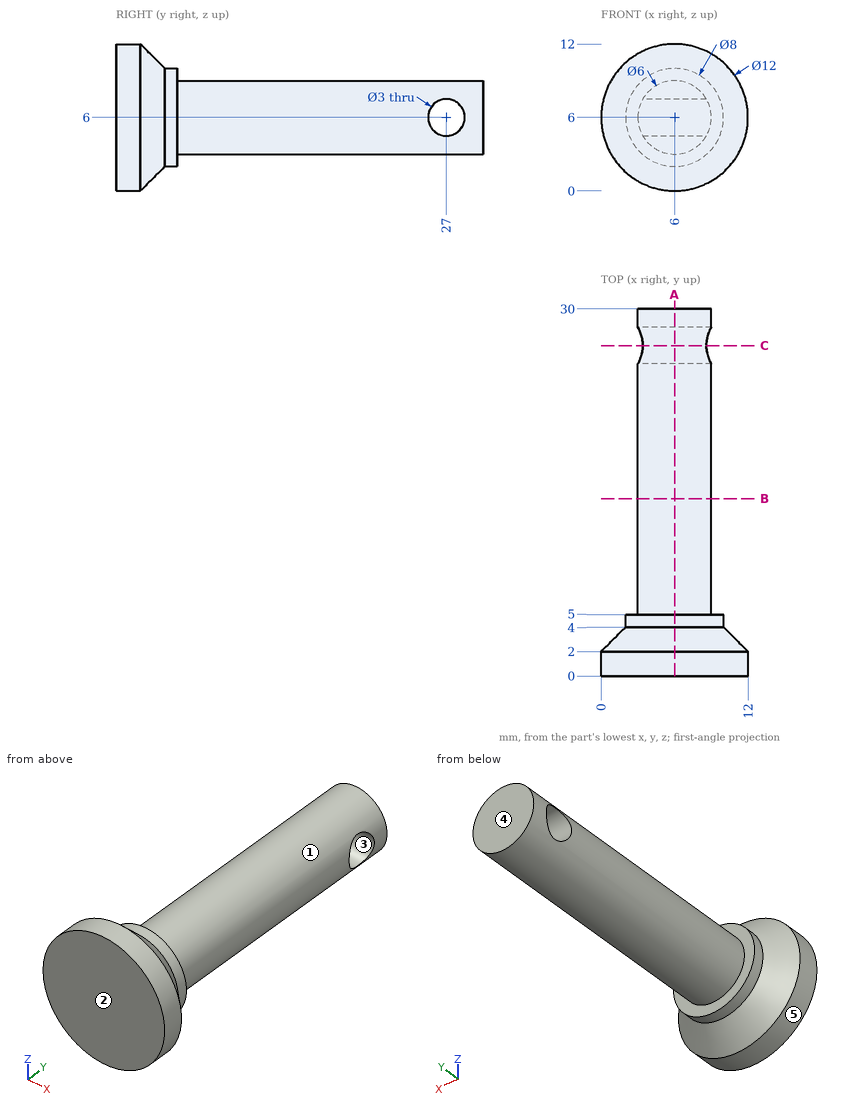
Here's the drawing with two shaded views (mm, measured from the low corner). I have some questions. A direction names the side the tool comes from. Coordinates: 2 decimals unless noted, no trailing zeros. Loops run counter-clockwise (first coordinate to the right, second up) from the corner with the lowest first, then second, coordinate; pieces in that order, holes last. Notation, with made-up numbers: (27, -27.5) - (42, -27.5) arc R22 cw to (42, -13.5) - close; hole circle Ø5 at (5, -31). An arc over 180 degrees is marked (long way). Answer as CSV lines item,"result". Start each with the question number.
1) Suppose I cut it at A-A (x = 6). Please give me the cut outline in (y, z).
2) Which directions (+Z, -Z, +X, -X, +Y, -Y) give clear straight access to the entire face, cutting with the end or side of a thin tool? Please do the marked faces 1 and 2.
3) Suppose I cut it at B-B (y = 14.5). Please give me the cut outline in (x, z).
4) Thinking about a two-plate mould opening in Z: for the marked faces 3, 4 and 5, which applies, pulls with the +Z half, pulls with the -Z half, needs draft (parallel to the pull), parting line crosses it, or undercut?
5) I need wall thicknesses on line 1 (Y direction, x = 5, z = 6); line 2 (Z direction, x = 6, y = 27); line 3 (Z direction, x = 3.5, y = 26). Which ranges of each line are inside material? Lowest first, please. Write a range as from..to.
6) For pin 1 (6 mm diameter, centred on x = 3, y = 26, fed in from +Z); pin 2 (2 mm diameter, centred on x = 8.5, y = 22.5, fed in from -Z); pin 3 (3 mm diameter, centred on y = 26.5, z = 10, fed in from -X), each with a flat end and sliding along its axis, tell me the tip position at first contact or that it passes through.
7) Suppose I cut it at C-C (y = 27). Please give me the cut outline in (x, z).
Check result:
1,outline,"(0, 0) - (2, 0) - (4, 2) - (5, 2) - (5, 3) - (30, 3) - (30, 9) - (5, 9) - (5, 10) - (4, 10) - (2, 12) - (0, 12) - close; hole circle Ø3 at (27, 6)"
2,face 1,"+Y"
2,face 2,"+Z, -Z, +X, -X, -Y"
3,outline,"circle Ø6 at (6, 6)"
4,face 3,"undercut"
4,face 4,"needs draft"
4,face 5,"parting line crosses it"
5,line 1,"y = 0..25.5, 28.5..30"
5,line 2,"z = 3..4.5, 7.5..9"
5,line 3,"z = 4.34..4.88, 7.12..7.66"
6,pin 1,"stops at z = 9"
6,pin 2,"stops at z = 3.4"
6,pin 3,"stops at x = 4.34"
7,outline,"(3.4, 4.5) arc R3 ccw to (8.6, 4.5) - close; (3.4, 7.5) - (8.6, 7.5) arc R3 ccw to start"
